Verification items for this drawing (mm, ordinates from the low corner). Coordinates: 2 decimals unless noted, no trailing zeros. Write each loop counter-clockwise with the first axis right and the second up, starting at its lowest first coordinate (ties: lowest second). Pieces come first, ordered by that corner, then holes. Notation, with made-up numbers: (-31.5, 12) -> (-12.5, 12) arc R25 cw to (-12.5, 30) -> close; hole circle Ø9 at (81, -27.75). An arc over 180 degrees is marked (long way). One line per item, written item: value. Start each with the question number.
1) Sectioned sample at C-C on x = 24. Enter the section's corners in (y, z).
2) Draft check along X on the marked faces 1, 2, 3 and 4. Enter one of: +X half, -X half, draft (parallel to the pull), parting line (faces both ways), or undercut.
3) Gauge pin test, flat ends, axial feed: P1, Ø1.5, axis at x = 41, z = 40.5, coming from the -Y side; P2, Ø3.5, axis at y = 27.5, z = 44, coming from the +X side; P3, Ø2.5, axis at y = 27.5, z = 44, coming from the -X side. Record the tip position at first contact, or that the pin passes through.
4) Sectioned sample at D-D on y = 41. Enter the section's corners in (x, z).
5) Sectioned sample at B-B on y = 34.5. Enter the section's corners in (x, z).
6) Sectioned sample at A-A on z = 42. Enter the section's corners in (x, y).
7) Scan lines: line 1 along Z through (x, y) = (39, 8); line 2 along Y through (x, z) = (27, 42); line 3 along Y through (x, z) = (25, 43). Record each from-to range of solid material in increasing order. Write a range as [from, to].
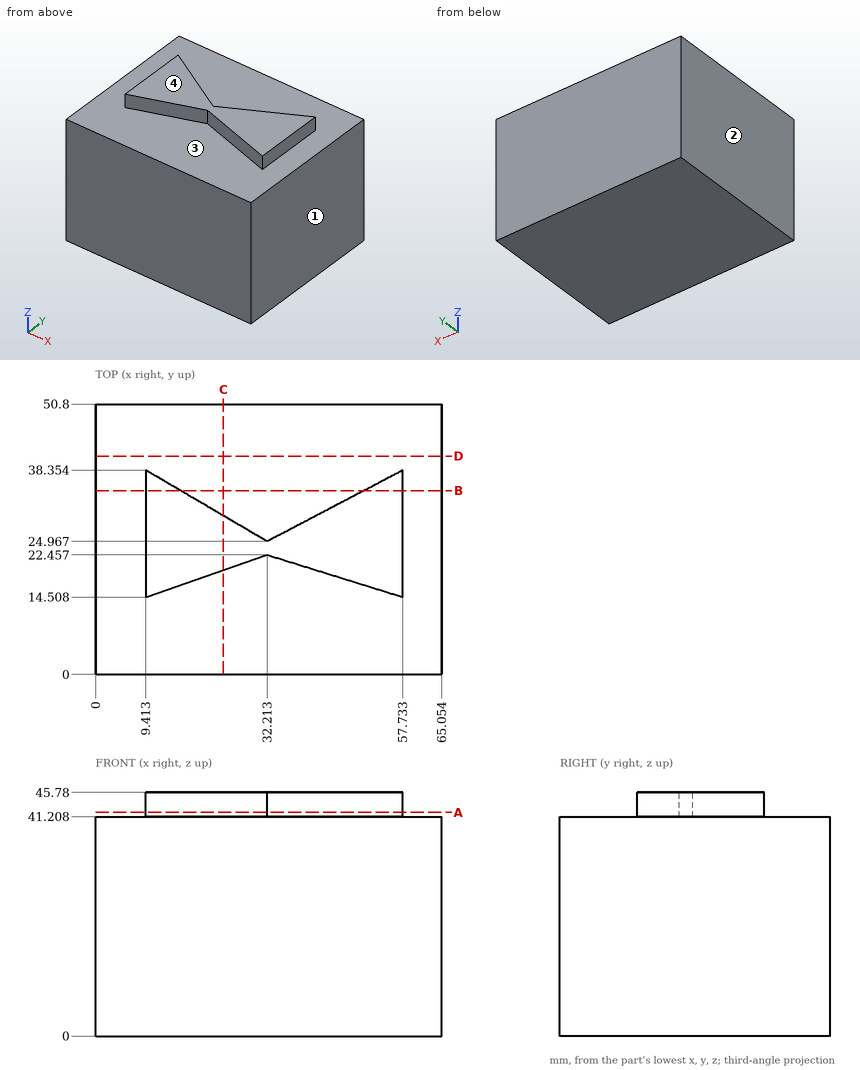
Answers:
1. outline: (0, 0) -> (50.8, 0) -> (50.8, 41.21) -> (29.79, 41.21) -> (29.79, 45.78) -> (19.59, 45.78) -> (19.59, 41.21) -> (0, 41.21) -> close
2. face 1: +X half
2. face 2: -X half
2. face 3: undercut
2. face 4: draft
3. P1: stops at y = 0
3. P2: stops at x = 57.73
3. P3: stops at x = 9.41
4. outline: (0, 0) -> (65.05, 0) -> (65.05, 41.21) -> (0, 41.21) -> close
5. outline: (0, 0) -> (65.05, 0) -> (65.05, 41.21) -> (57.73, 41.21) -> (57.73, 45.78) -> (50.39, 45.78) -> (50.39, 41.21) -> (15.98, 41.21) -> (15.98, 45.78) -> (9.41, 45.78) -> (9.41, 41.21) -> (0, 41.21) -> close
6. outline: (9.41, 14.51) -> (32.21, 22.46) -> (57.73, 14.51) -> (57.73, 38.35) -> (32.21, 24.97) -> (9.41, 38.35) -> close
7. line 1: z = [0, 41.21]
7. line 2: y = [20.64, 28.03]
7. line 3: y = [19.94, 29.2]
